Check sheet for the drawn part. Datum: minimum x, y, z corner. Units: mm. A direction names the side the tool comes from. Give positions to 0.01 mm unless a question says otherwise; leave off trailing zeros. Order: outer loops, then holes, each group sorted by start corner. A loop starts at its lowest first (then second) coordinate and runs counter-clockwise, first axis right, second up.
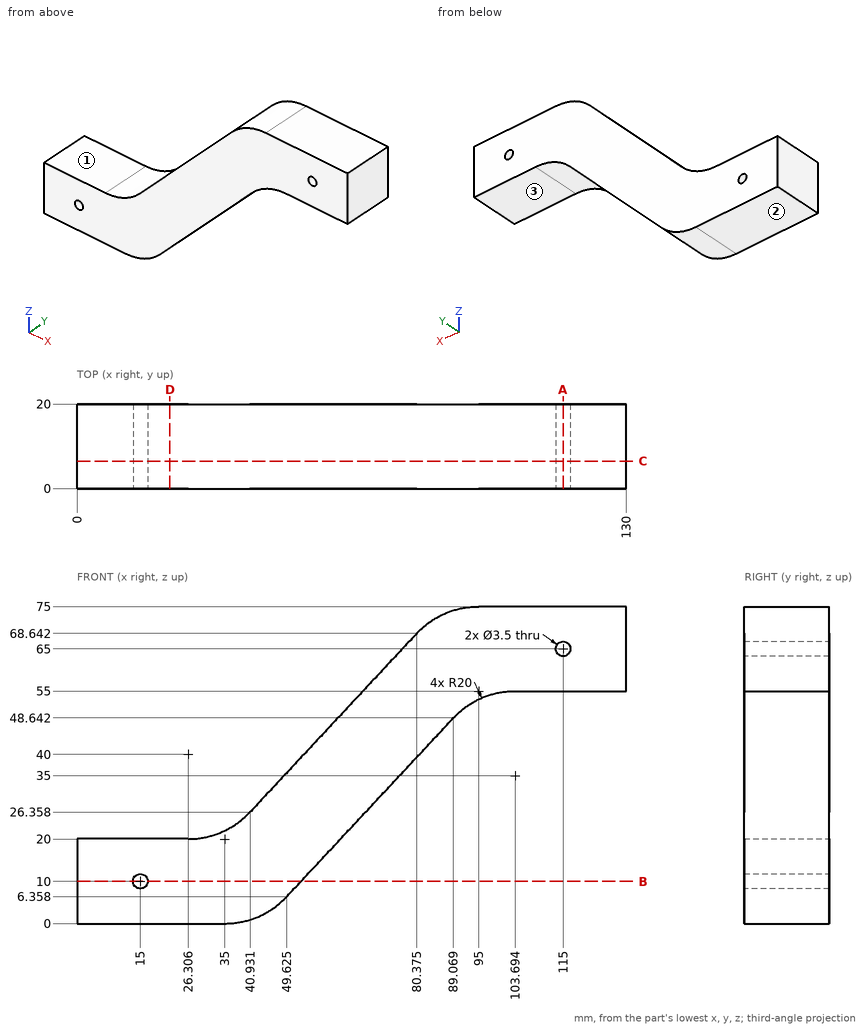
Item 1: Sectioned sample at D-D (x = 22). Enter the section's corners in (y, z), and give its area (3 significant figures).
Reported:
outline: (0, 0) - (20, 0) - (20, 20) - (0, 20) - close
area: 400 mm2
Item 2: Sectioned sample at A-A (x = 115). Enter the section's corners in (y, z).
Reported:
outline: (0, 55) - (20, 55) - (20, 63.25) - (0, 63.25) - close; (0, 66.75) - (20, 66.75) - (20, 75) - (0, 75) - close
Item 3: Gauge pin test, flat ends, axial feed: pin 1 (6 mm diameter, centred on x = 11.5, y = 14, fed in from +Z); pin 2 (3 mm diameter, centred on x = 88.5, z = 55.5, fed in from -Y); pin 3 (6 mm diameter, centred on y = 14, z = 28.5, fed in from -X); pin 4 (1 mm diameter, centred on x = 60.5, y = 10, fed in from -Z). Record the tip position at first contact, or that the pin passes through.
Reported:
pin 1: stops at z = 20
pin 2: stops at y = 0
pin 3: stops at x = 40.08
pin 4: stops at z = 17.48
Item 4: Sectioned sample at B-B (z = 10). Enter the section's corners in (x, y).
Reported:
outline: (0, 0) - (13.25, 0) - (13.25, 20) - (0, 20) - close; (16.75, 0) - (53.02, 0) - (53.02, 20) - (16.75, 20) - close
Item 5: Scan lines: L1, parallel to Z at x = 15, y = 14.5; L2, parallel to Z at x = 115, y = 5.25; L3, parallel to Z at x = 11, y = 1. Record each from-to range of solid material in increasing order.
Reported:
L1: z = 0 to 8.25, 11.75 to 20
L2: z = 55 to 63.25, 66.75 to 75
L3: z = 0 to 20
Item 6: Set-up check for the marked faces 1, 2 and 3: record each of +Z, -Z, +X, -X, +Y, -Y from which the full face is reachable in a straight line by a thin tool's end or side.
Reported:
face 1: +Z, -X, +Y, -Y
face 2: -Z, +X, -X, +Y, -Y
face 3: -Z, +X, +Y, -Y
Item 7: Sectioned sample at C-C (y = 6.5). Give the number of separate pieces and of enclosed holes in the cut face, and give its area (3 significant figures).
Reported:
separate pieces: 1
enclosed holes: 2
area: 3,060 mm2
